from build123d import *

# Parameters (mm, degrees)
SKETCH_1_W          = 75
SKETCH_1_H          = 45
SKETCH_1_R          = 3
EXTRUDE_1_DEPTH     = 5
SKETCH_2_W          = 5
SKETCH_2_H          = 5.5
SKETCH_2_W_2        = 5.5
CUT_EXTRUDE_1_DEPTH = 5
FILLET_1_R          = 5


with BuildPart() as part:
    # 草图1 → 凸台-拉伸1 (new body)
    with BuildSketch(Plane.XY):
        with Locations((37.5, -22.5)):
            Rectangle(SKETCH_1_W, SKETCH_1_H)
        with Locations((21.13500001, -28.900000005)):
            Circle(SKETCH_1_R, mode=Mode.SUBTRACT)
        with Locations((56.59, -28.4)):
            Circle(SKETCH_1_R, mode=Mode.SUBTRACT)
    extrude(amount=EXTRUDE_1_DEPTH)

    # 草图2 → 切除-拉伸1 (cut)
    with BuildSketch(Plane.XY.offset(5)):
        Polygon((40.5, -8.5), (40.5, -3), (37.5, -3), (35, -3), (35, -8.5), align=None)
        with Locations((60.75, -5.75)):
            Rectangle(SKETCH_2_W, SKETCH_2_H)
        with Locations((14.5, -5.75)):
            Rectangle(SKETCH_2_W_2, SKETCH_2_H)
    extrude(amount=-CUT_EXTRUDE_1_DEPTH, mode=Mode.SUBTRACT)

    # 圆角1
    fillet_1_edges = [part.edges().sort_by_distance(p)[0] for p in [
        (0, 0, 2.5),
        (75, 0, 2.5),
        (75, -45, 2.5),
        (0, -45, 2.5),
    ]]
    fillet(fillet_1_edges, radius=FILLET_1_R)


solid = part.part
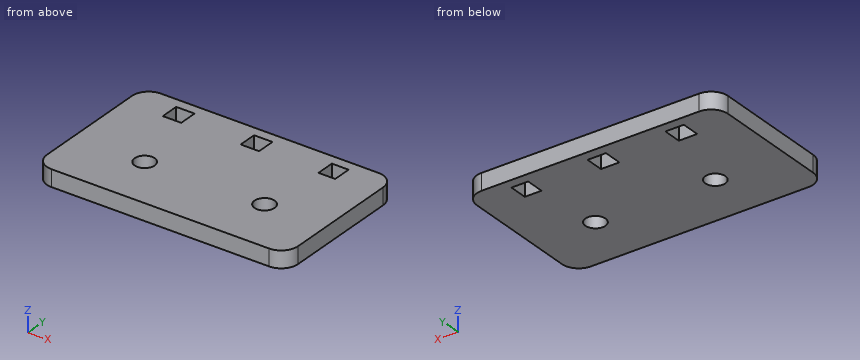
Could you check a few things on this model? Use its own coordinates, in mm. Round coordinates to 2 decimals unless told otherwise and drop trailing zeros. Loops run counter-clockwise (first coordinate to the right, second up) from the corner with the lowest first, then second, coordinate; pieces in that order, holes last. Notation, with made-up numbers: (56.5, -30) -> (76.5, -30) arc R24 cw to (76.5, -5) -> close; hole circle Ø10 at (-15.5, -12). An arc over 180 degrees is marked (long way). Use CSV: the item, a comma, the result in double quotes.
(1) Suppose I cut it at D-D on x = 15. Write out the boundary of the cut face in (y, z).
Return value:
outline,"(-45, 0) -> (-8.5, 0) -> (-8.5, 5) -> (-45, 5) -> close; (-3, 0) -> (0, 0) -> (0, 5) -> (-3, 5) -> close"
(2) Suppose I cut it at A-A on x = 56.59. Write out the boundary of the cut face in (y, z).
Return value:
outline,"(-45, 0) -> (-31.4, 0) -> (-31.4, 5) -> (-45, 5) -> close; (-25.4, 0) -> (0, 0) -> (0, 5) -> (-25.4, 5) -> close"
(3) Suppose I cut it at C-C on z = 3.95. Write out the boundary of the cut face in (x, y) (3 decimals), plus the area to 3 significant figures.
Return value:
outline,"(0, -40) arc R5 ccw to (5, -45) -> (70, -45) arc R5 ccw to (75, -40) -> (75, -5) arc R5 ccw to (70, 0) -> (5, 0) arc R5 ccw to (0, -5) -> close; hole (11.75, -8.5) -> (17.25, -8.5) -> (17.25, -3) -> (11.75, -3) -> close; hole circle Ø6 at (21.135, -28.9); hole (35, -8.5) -> (40.5, -8.5) -> (40.5, -3) -> (35, -3) -> close; hole circle Ø6 at (56.59, -28.4); hole (58.25, -8.5) -> (63.25, -8.5) -> (63.25, -3) -> (58.25, -3) -> close"
area,"3,210 mm²"
(4) If I drill on probe 1 along X at (y, z) = (-7.5, 2.55); probe 2 along Y at (x, z) = (13, 4.1); probe 3 along Y at (x, z) = (56.59, 2.05), over which ranges is the centre line in solid material (lowest first)? Write a range as [from, to].
Return value:
probe 1,"x = [0, 11.75], [17.25, 35], [40.5, 58.25], [63.25, 75]"
probe 2,"y = [-45, -8.5], [-3, 0]"
probe 3,"y = [-45, -31.4], [-25.4, 0]"
(5) Will this pin go through, and if not, where does the flat tip stop? pin 1 Ø8 at (x, y) = (21.135, -28.9) entering from -Z.
Return value:
pin 1,"stops at z = 0"
(6) Suppose I cut it at B-B on y = -6.5. Write out the boundary of the cut face in (x, z).
Return value:
outline,"(0, 0) -> (11.75, 0) -> (11.75, 5) -> (0, 5) -> close; (17.25, 0) -> (35, 0) -> (35, 5) -> (17.25, 5) -> close; (40.5, 0) -> (58.25, 0) -> (58.25, 5) -> (40.5, 5) -> close; (63.25, 0) -> (75, 0) -> (75, 5) -> (63.25, 5) -> close"
